Autodesk Inventor part; units mm, degrees
ref_plane "YZ Plane" through (0, 0, 0) normal (1, 0, 0) x (0, 1, 0)
ref_plane "XZ Plane" through (0, 0, 0) normal (0, 1, 0) x (-1, 0, 0)
ref_plane "XY Plane" through (0, 0, 0) normal (0, 0, 1) x (1, 0, 0)
sketch "Szkic1" plane through (0, 0, 0) normal (1, 0, 0) x (0, 1, 0)
  point P0 (0, 0)
sketch "Szkic2" plane through (0, 0, 0) normal (1, 0, 0) x (0, 1, 0)
  point P0 (0, 0)
sketch "Szkic3" plane through (0, 0, 0) normal (1, 0, 0) x (0, 1, 0)
  line L0 (0, 19.7455) -> (50, 19.7455)
  line L1 (50, 19.7455) -> (50, 3.5455)
  line L2 (50, 3.5455) -> (43.564, -2.8878)
  line L3 (43.564, -2.8878) -> (43.564, -138.8878)
  line L4 (43.564, -138.8878) -> (50, -145.3212)
  line L5 (50, -145.3212) -> (50, -161.5212)
  line L6 (50, -161.5212) -> (0, -161.5212)
  line L7 (0, 19.7455) -> (0, -161.5212)
  point P0 (0, 0)
  dimension "d0" = 50
  dimension "d1" = 16.2
  dimension "d2" = 9.1
  dimension "d3" = 136
  dimension "d4" = 9.1
  dimension "d5" = 16.2
revolve "Obrót1" add sketch "Szkic3" angle 360 about axis through (0, 0, 19.7455) along (0, 0, -1)
sketch "Szkic4" plane through (0, 0, -161.5212) normal (0, 0, -1) x (-1, 0, 0)
  line L0 (0, 0) -> (40, 0)
  line L1 (0, 0) -> (0, -40)
  line L2 (0, 0) -> (-40, 0)
  line L3 (0, 0) -> (0, 40)
  dimension "d7" = 40
  dimension "d8" = 40
  dimension "d9" = 40
  dimension "d10" = 40
hole "Otwór1" at (0, 40, -161.5212) at (-40, 0, -161.5212) at (0, -40, -161.5212) at (40, 0, -161.5212) direction (0, 0, 1) diameter 5 depth 18.5 tip angle 118
sketch "Szkic5" plane through (0, 0, 19.7455) normal (0, 0, 1) x (1, 0, 0)
  circle A0 centre (40, 0) radius 2.5
  line L0 (0, 0) -> (40, 0)
  circle A1 centre (0, -40) radius 2.5
  line L1 (0, 0) -> (0, -40)
  circle A2 centre (0, 0) radius 50
  circle A3 centre (-40, 0) radius 2.5
  line L2 (0, 0) -> (-40, 0)
  circle A4 centre (0, 40) radius 2.5
  line L3 (0, 0) -> (0, 40)
hole "Otwór2" at (-40, 0, 19.7455) at (0, 40, 19.7455) at (40, 0, 19.7455) at (0, -40, 19.7455) direction (0, 0, -1) diameter 5 depth 18.5 tip angle 118
sketch "Szkic6" plane through (0, 0, 19.7455) normal (0, 0, 1) x (1, 0, 0)
  line L0 (0, 0) -> (0, 50)
  circle A0 centre (0, 0) radius 50
hole "Otwór3" at (0, 0, 19.7455) direction (0, 0, -1) diameter 70 end through all
sketch "Szkic7" plane through (0, 0, 19.7455) normal (0, 0, 1) x (1, 0, 0)
  point P0 (0, 0)
properties part number "korpus"
Can you work these out from the model? Positions are in its coordinate system, mm. A direction names the side the tool comes from. Round coordinates to 2 decimals unless told otherwise and drop trailing zeros. Loops run counter-clockwise (first coordinate to the right, second up) from the corner with the lowest first, then second, coordinate; pieces in that order, holes last. Notation, with made-up numbers: (66, 50) -> (80, 50) arc R26 cw to (80, 71) -> close; hole circle Ø2 at (-29, -25). An arc over 180 degrees is marked (long way). Answer in a Markdown table with one row per item.
Item 1: Will these pins go through, and if not, where does the flat tip stop? P1, Ø5, axis at x = -4, z = -48, coming from the +Y side; P2, Ø4, axis at x = 0, y = 40, coming from the +Z side; P3, Ø2, axis at x = -35.5, y = 37, coming from the +Z side; P4, Ø12, axis at y = -37, z = -47, coming from the -X side.
Answer block:
| item | result |
|---|---|
| P1 | y = 43.54 |
| P2 | z = 0.95 |
| P3 | through |
| P4 | x = -30.61 |
Item 2: Suppose I cut it at B-B, the plane z = -119.5. List the corners of the cut face in (x, y) for me, plus the area to 3 significant figures.
Answer block:
| item | result |
|---|---|
| outline | circle Ø87.13 at (0, 0); hole circle Ø70 at (0, 0) |
| area | 2,110 mm² |
Item 3: On a 3-axis mill with a long thin cutter (end or side, diameter ignored), from which of +Z, -Z, +X, -X, +Y, -Y can I reach the whole of each face in a straight line? I mean faces 1 (the conical face through (42.921, -9.531, -2.485)), 2 (the cylindrical face through (-37.56, 0.54, 10.37)), 3 (the cylindrical face through (-37.56, -0.54, -152.14)), 4 (the cylindrical face through (15.02, 47.69, -153.53)). Say none if no direction works.
Answer block:
| item | result |
|---|---|
| face 1 | none |
| face 2 | +Z |
| face 3 | -Z |
| face 4 | +Z, -Z |
Item 4: If I drill on probe 1 along X at (y, z) = (0, -147.75); probe 2 along X at (y, z) = (-1.5, -114); probe 3 along Y at (x, z) = (13, -86), over which ranges is the centre line in solid material (lowest first)?
Answer block:
| item | result |
|---|---|
| probe 1 | -50 to -42.5, -37.5 to -35, 35 to 37.5, 42.5 to 50 |
| probe 2 | -43.54 to -34.97, 34.97 to 43.54 |
| probe 3 | -41.58 to -32.5, 32.5 to 41.58 |
Item 5: We'd pull the mould along Y, two halves only. Please class faces 5 (the cylindrical face through (13.09, 41.55, -71.84)), 6 (the cylindrical face through (42.44, 0.54, 10.37)), 7 (the flat face through (-10, -34, -161.521)): released by +Y, released by -Y, zero draft, split by the parting line, or undercut.
Answer block:
| item | result |
|---|---|
| face 5 | split by the parting line |
| face 6 | undercut |
| face 7 | zero draft |
Item 6: Suppose I cut it at A-A, the plane z = 9. List the corners of the cut face in (x, y) for me.
Answer block:
| item | result |
|---|---|
| outline | circle Ø100 at (0, 0); hole circle Ø5 at (-40, 0); hole circle Ø70 at (0, 0); hole circle Ø5 at (0, -40); hole circle Ø5 at (0, 40); hole circle Ø5 at (40, 0) |
